```python
from build123d import *

# Parameters (mm, degrees)
ESQUISSE1_W        = 10
ESQUISSE1_H        = 10
BOSS_EXTRU_1_DEPTH = 42


with BuildPart() as part:
    # Esquisse1 → Boss.-Extru.1 (new body)
    with BuildSketch(Plane(origin=(0, 0, 0), x_dir=(1, 0, 0), z_dir=(0, 1, 0))):
        Polygon((0, -21.2), (0, -31.2), (17.87, -31.2), (17.87, 48.8), (-10, 48.8), (-80, 18.8), (-80, -31.2), (-10, -31.2), (-10, -21.2), align=None)
        with Locations((-5, 26.2)):
            Rectangle(ESQUISSE1_W, ESQUISSE1_H, mode=Mode.SUBTRACT)
    extrude(amount=BOSS_EXTRU_1_DEPTH)


solid = part.part
```
Build history of the part. All positions in model axes, mm. A direction names the side the tool comes from. Give positions to 0.01 mm unless a question says otherwise; leave off trailing zeros. Loops run counter-clockwise (first coordinate to the right, second up) from the corner with the lowest first, then second, coordinate; pieces in that order, holes last.
Item 1: Slice it at D-D, the plane x = -21. List the corners of the cut face in (y, z), and give its area (3 significant figures).
Answers follow:
outline: (0, -44.09) - (42, -44.09) - (42, 31.2) - (0, 31.2) - close
area: 3,160 mm2
Item 2: Flat gauge pins, fed straight in: pin 1 (8 mm diameter, centred on x = -28.5, y = 10.5, fed in from -Z); pin 2 (5 mm diameter, centred on y = 24, z = -28.5, fed in from -X); pin 3 (3 mm diameter, centred on x = -5, y = 26, fed in from +Z). Where does each tip first touch, or does it go through?
Answers follow:
pin 1: stops at z = -42.59
pin 2: stops at x = -63.2
pin 3: stops at z = 21.2
Item 3: Slice it at C-C, the plane z = -25. List the corners of the cut face in (x, y), and give its area (3 significant figures).
Answers follow:
outline: (-65.53, 0) - (-10, 0) - (-10, 42) - (-65.53, 42) - close; (0, 0) - (17.87, 0) - (17.87, 42) - (0, 42) - close
area: 3,080 mm2
Item 4: Slice it at A-A, the plane x = -4. List the corners of the cut face in (y, z), and give its area (3 significant figures).
Answers follow:
outline: (0, -48.8) - (42, -48.8) - (42, -31.2) - (0, -31.2) - close; (0, -21.2) - (42, -21.2) - (42, 21.2) - (0, 21.2) - close
area: 2,520 mm2
Item 5: Which spindle directions (+Z, -Z, +X, -X, +Y, -Y) get a long thin tool onto all of the face, cutting with end or side? Do faces 5 (the face through (-10, 21, 26)), 6 (the face through (17.87, 21, -8)), 7 (the face through (0, 21, -26)). Say none if no direction does.
Answers follow:
face 5: +Z, +Y, -Y
face 6: +Z, -Z, +X, +Y, -Y
face 7: +Y, -Y
Item 6: Slice it at B-B, the plane y = 15. List the corners of the cut face in (x, z).
Answers follow:
outline: (-80, -18.8) - (-10, -48.8) - (17.87, -48.8) - (17.87, 31.2) - (0, 31.2) - (0, 21.2) - (-10, 21.2) - (-10, 31.2) - (-80, 31.2) - close; hole (-10, -31.2) - (0, -31.2) - (0, -21.2) - (-10, -21.2) - close
Item 7: Pull direction Z, two halves, no side cores. Call faces 1 (the face through (-5, 21, -21.2)), 2 (the face through (-10, 21, -26)), 3 (the face through (0, 21, 26)), 4 (the face through (-5, 21, 21.2)): released by +Z, released by -Z, zero draft, split by the parting line, or undercut.
Answers follow:
face 1: undercut
face 2: undercut
face 3: zero draft
face 4: released by +Z
Item 8: Drill centre lines: line 1 (Z direction, x = -1.5, y = 10); line 2 (X direction, y = 25.5, z = -36.5); line 3 (Z direction, x = -41.5, y = 36). Where is each one in solid material? Low to high.
Answers follow:
line 1: z = -48.8 to -31.2, -21.2 to 21.2
line 2: x = -38.7 to 17.87
line 3: z = -35.3 to 31.2
